Can you work these out from the model? Positions are in its coordinate system, mm. Face numbers are marked on the shaded views. A direction names the side the tool comes from. Give positions to 0.01 mm unless a question says otherwise; leave off trailing zeros. Loops run counter-clockwise (first coordinate to the right, second up) from the corner with the lowest first, then second, coordinate; pieces in that order, holes last. Notation, with made-up numbers: (36, -20.5) -> (76, -20.5) arc R8 cw to (76, -8.5) -> close; hole circle Ø5 at (-2, -26). An arc over 180 degrees is marked (long way). Return JSON: item names as keys, results as strings. Group by question number.
Q1. Will these pins go through, and if not, where does the flat tip stop? pin 1 (8 mm diameter, centred on y = 4, z = 89, fed in from -X); pin 2 (11 mm diameter, centred on y = 2.5, z = -90.5, fed in from +X); pin 3 (3 mm diameter, centred on x = -93.5, y = 6.5, fed in from -Z); pin 4 (2.5 mm diameter, centred on x = -14.14, z = -14.14, fed in from +Y).
Q2. Suppose I cut it at B-B, the plane z = 0. Please give me the cut outline in (x, y), and give its area (3 significant figures).
Q3. I need wall thicknesses on line 1 along X through (y, z) = (-1, -13.5); line 2 along Z through (x, y) = (73, 9.25); line 3 along Y through (x, z) = (-8, -63). Which ranges of each line are inside material? Lowest first, please. Write a range as [from, to].
Q4. Suppose I cut it at C-C, the plane x = -39. Count the separate pieces of the cut face and the enclosed holes in it, and give its area (3 significant figures).
Q5. Which directions (+Z, -Z, +X, -X, +Y, -Y) give clear straight access to the entire face, cutting with the end or side of a thin tool? Please do the marked faces 1 and 2.
Q6. Suppose I cut it at A-A, the plane x = 0. Please give me the cut outline in (y, z).
```python
from build123d import *

# Parameters (mm, degrees)
SKIZZE1_R                       = 100
AUFSATZ_LINEAR_AUSTRAGEN1_DEPTH = 10
SKIZZE2_W                       = 15
SKIZZE2_H                       = 15
SCHNITT_LINEAR_AUSTRAGEN1_DEPTH = 142.774468788
SKIZZE3_R                       = 52.5
AUFSATZ_LINEAR_AUSTRAGEN2_DEPTH = 10
FASE1_SIZE                      = 2
SKIZZE4_R                       = 2.1
SCHNITT_LINEAR_AUSTRAGEN2_DEPTH = 143.434195332
FASE2_SIZE                      = 3


with BuildPart() as part:
    # Skizze1 → Aufsatz-Linear austragen1 (new body)
    with BuildSketch(Plane(origin=(0, 0, 0), x_dir=(1, 0, 0), z_dir=(0, 1, 0))):
        with Locations(Location((0, 0, 0), (0, 0, 270))):
            Circle(SKIZZE1_R)
    extrude(amount=AUFSATZ_LINEAR_AUSTRAGEN1_DEPTH)

    # Skizze2 → Schnitt-Linear austragen1 (cut, through all)
    with BuildSketch(Plane(origin=(0, 10, 0), x_dir=(1, 0, 0), z_dir=(0, 1, 0))):
        Polygon((77.362159322, -36.004809472), (90.352540378, -43.504809472), (82.852540378, -56.495190528), (69.862159322, -48.995190528), align=None)
        with Locations((92.5, 0)):
            Rectangle(SKIZZE2_W, SKIZZE2_H)
        Polygon((48.995190528, -69.862159322), (56.495190528, -82.852540378), (43.504809472, -90.352540378), (36.004809472, -77.362159322), align=None)
        with Locations((0, -92.5)):
            Rectangle(SKIZZE2_W, SKIZZE2_H)
        Polygon((-36.004809472, -77.362159322), (-43.504809472, -90.352540378), (-56.495190528, -82.852540378), (-48.995190528, -69.862159322), align=None)
        Polygon((-69.862159322, -48.995190528), (-82.852540378, -56.495190528), (-90.352540378, -43.504809472), (-77.362159322, -36.004809472), align=None)
        with Locations((-92.5, 0)):
            Rectangle(SKIZZE2_W, SKIZZE2_H)
        Polygon((-77.362159322, 36.004809472), (-90.352540378, 43.504809472), (-82.852540378, 56.495190528), (-69.862159322, 48.995190528), align=None)
        Polygon((-48.995190528, 69.862159322), (-56.495190528, 82.852540378), (-43.504809472, 90.352540378), (-36.004809472, 77.362159322), align=None)
        with Locations((0, 92.5)):
            Rectangle(SKIZZE2_W, SKIZZE2_H)
        Polygon((36.004809472, 77.362159322), (43.504809472, 90.352540378), (56.495190528, 82.852540378), (48.995190528, 69.862159322), align=None)
        Polygon((69.862159322, 48.995190528), (82.852540378, 56.495190528), (90.352540378, 43.504809472), (77.362159322, 36.004809472), align=None)
    extrude(amount=-SCHNITT_LINEAR_AUSTRAGEN1_DEPTH, mode=Mode.SUBTRACT)

    # Skizze3 → Aufsatz-Linear austragen2 (add)
    with BuildSketch(Plane.XZ):
        with Locations(Location((0, 0, 0), (0, 0, 90))):
            Circle(SKIZZE3_R)
    extrude(amount=AUFSATZ_LINEAR_AUSTRAGEN2_DEPTH)

    # Fase1
    fase1_edges = [part.edges().sort_by_distance(p)[0] for p in [
        (0, -10, -52.5),
    ]]
    chamfer(fase1_edges, length=FASE1_SIZE)

    # Skizze4 → Schnitt-Linear austragen2 (cut, through all)
    with BuildSketch(Plane(origin=(0, 10, 0), x_dir=(1, 0, 0), z_dir=(0, 1, 0))):
        with Locations(Location((-14.142135624, 14.142135624, 0), (0, 0, 270))):
            Circle(SKIZZE4_R)
        with Locations(Location((14.142135624, 14.142135624, 0), (0, 0, 270))):
            Circle(SKIZZE4_R)
        with Locations(Location((14.142135624, -14.142135624, 0), (0, 0, 270))):
            Circle(SKIZZE4_R)
        with Locations(Location((-14.142135624, -14.142135624, 0), (0, 0, 270))):
            Circle(SKIZZE4_R)
    extrude(amount=-SCHNITT_LINEAR_AUSTRAGEN2_DEPTH, mode=Mode.SUBTRACT)

    # Fase2
    fase2_edges = [part.edges().sort_by_distance(p)[0] for p in [
        (-14.142135624, 10, 12.042135624),
        (14.142135624, 10, 12.042135624),
        (14.142135624, 10, -16.242135624),
        (-14.142135624, 10, -16.242135624),
    ]]
    chamfer(fase2_edges, length=FASE2_SIZE)


solid = part.part
```
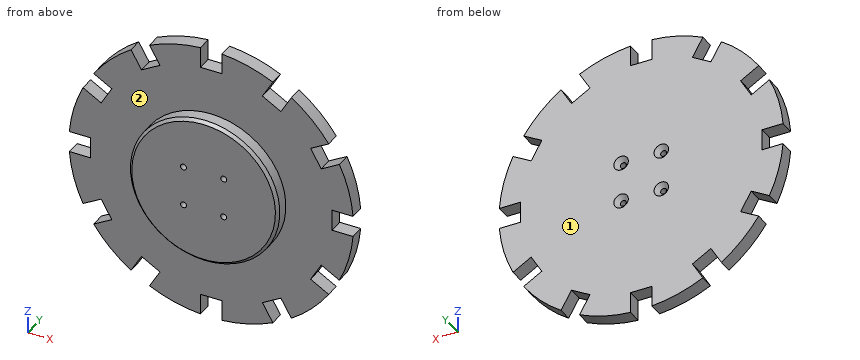
Ans:
{
 "1": {"pin 1": "stops at x = -43.36", "pin 2": "stops at x = 43.36", "pin 3": "stops at z = -39.19", "pin 4": "passes through"},
 "2": {"outline": "(-85, 0) -> (-52.5, 0) -> (-52.5, -8) -> (-50.5, -10) -> (50.5, -10) -> (52.5, -8) -> (52.5, 0) -> (85, 0) -> (85, 10) -> (-85, 10) -> close", "area": "2,750 mm^2"},
 "3": {"line 1": "x = [-50.73, -16.14], [-12.14, 12.14], [16.14, 50.73]", "line 2": "z = [-68.34, -50.81], [-43.56, 43.56], [50.81, 68.34]", "line 3": "y = [0, 10]"},
 "4": {"separate pieces": "3", "enclosed holes": "0", "area": "2,400 mm^2"},
 "5": {"face 1": "+Z, -Z, +X, -X, +Y", "face 2": "-Y"},
 "6": {"outline": "(-10, -50.5) -> (-8, -52.5) -> (0, -52.5) -> (0, -85) -> (10, -85) -> (10, 85) -> (0, 85) -> (0, 52.5) -> (-8, 52.5) -> (-10, 50.5) -> close"}
}
